Can you work these out from the model? Positions are in its coordinate system, mm. A direction names the side the tool comes from. Give positions to 0.01 mm unless a question says otherwise; leave off trailing zeros. Write each loop counter-clockwise with the first axis right and the second up, starting at its lowest first coordinate (ties: lowest second). Pieces come first, ordered by that corner, then holes.
```python
from build123d import *

# Parameters (mm, degrees)
SKETCH_R        = 2
SKETCH_R_2      = 8.25
SKETCH_R_3      = 3
SKETCH_R_4      = 1.5
PAD_DEPTH       = 10
SKETCH004_R     = 3.5
SKETCH004_R_2   = 2.8
POCKET_DEPTH    = 4
POCKET001_DEPTH = 2.5
SKETCH006_R     = 5
POCKET002_DEPTH = 6


with BuildPart() as part:
    # Sketch → Pad (new body)
    with BuildSketch(Plane.XY):
        with BuildLine():
            Line((0, 0), (0, 34))
            ThreePointArc((0, 34), (-1.757359, 38.242641), (-6, 40))
            Line((-19, 40), (-6, 40))
            ThreePointArc((-25, 46), (-23.242641, 41.757359), (-19, 40))
            Line((-25, 54), (-25, 46))
            ThreePointArc((-19, 60), (-23.242641, 58.242641), (-25, 54))
            Line((-19, 60), (54, 60))
            ThreePointArc((60, 54), (58.242641, 58.242641), (54, 60))
            Line((60, 54), (60, 46))
            ThreePointArc((60, 46), (61.757359, 41.757359), (66, 40))
            Line((66, 40), (89, 40))
            ThreePointArc((95, 34), (93.242641, 38.242641), (89, 40))
            Line((95, 34), (95, 26))
            ThreePointArc((95, 26), (96.757359, 21.757359), (101, 20))
            Line((101, 20), (134, 20))
            ThreePointArc((140, 14), (138.242641, 18.242641), (134, 20))
            Line((140, 14), (140, 0))
            Line((140, 0), (0, 0))
        make_face()
        with Locations((10, 10)):
            Circle(SKETCH_R, mode=Mode.SUBTRACT)
        with Locations((33.5, 39)):
            Circle(SKETCH_R_2, mode=Mode.SUBTRACT)
        with Locations((81.5, 26)):
            Circle(SKETCH_R_3, mode=Mode.SUBTRACT)
        with Locations((130, 10)):
            Circle(SKETCH_R, mode=Mode.SUBTRACT)
        with Locations((40, 10)):
            Circle(SKETCH_R_4, mode=Mode.SUBTRACT)
        with Locations((90, 10)):
            Circle(SKETCH_R_4, mode=Mode.SUBTRACT)
        with Locations((-15.5, 50)):
            Circle(SKETCH_R_3, mode=Mode.SUBTRACT)
    extrude(amount=PAD_DEPTH)

    # Sketch004 → Pocket (cut)
    with BuildSketch(Plane.XY):
        with Locations((10, 10)):
            Circle(SKETCH004_R)
        with Locations((40, 10)):
            Circle(SKETCH004_R_2)
        with Locations((130, 10)):
            Circle(SKETCH004_R)
        with Locations((90, 10)):
            Circle(SKETCH004_R_2)
    extrude(amount=POCKET_DEPTH, mode=Mode.SUBTRACT)

    # Sketch005 (on Face5 of Pocket) → Pocket001 (cut)
    with BuildSketch(Plane.XY.offset(10)):
        Polygon((40, 6.8), (42.771281, 8.4), (42.771281, 11.6), (40, 13.2), (37.228719, 11.6), (37.228719, 8.4), align=None)
        Polygon((90, 6.8), (92.771281, 8.4), (92.771281, 11.6), (90, 13.2), (87.228719, 11.6), (87.228719, 8.4), align=None)
    extrude(amount=-POCKET001_DEPTH, mode=Mode.SUBTRACT)

    # Sketch006 (on Face5 of Pocket) → Pocket002 (cut)
    with BuildSketch(Plane.XY.offset(10)):
        with Locations((81.5, 26)):
            Circle(SKETCH006_R)
        with Locations((-15.5, 50)):
            Circle(SKETCH006_R)
    extrude(amount=-POCKET002_DEPTH, mode=Mode.SUBTRACT)


solid = part.part
```
1) Suppose I cut it at B-B on y = 50. Write out the boundary of the cut face in (x, z).
Values follow:
outline: (-25, 0) - (-18.5, 0) - (-18.5, 4) - (-20.5, 4) - (-20.5, 10) - (-25, 10) - close; (-12.5, 0) - (60, 0) - (60, 10) - (-10.5, 10) - (-10.5, 4) - (-12.5, 4) - close
2) Suppose I cut it at D-D on y = 10. State how many separate pieces and enclosed holes the cut face has, plus the area to 3 significant figures.
Values follow:
separate pieces: 5
enclosed holes: 0
area: 1,200 mm2
3) Suppose I cut it at C-C on z = 1.75. Write out the boundary of the cut face in (x, y).
Values follow:
outline: (-25, 46) arc R6 ccw to (-19, 40) - (-6, 40) arc R6 cw to (0, 34) - (0, 0) - (140, 0) - (140, 14) arc R6 ccw to (134, 20) - (101, 20) arc R6 cw to (95, 26) - (95, 34) arc R6 ccw to (89, 40) - (66, 40) arc R6 cw to (60, 46) - (60, 54) arc R6 ccw to (54, 60) - (-19, 60) arc R6 ccw to (-25, 54) - close; hole circle Ø6 at (-15.5, 50); hole circle Ø7 at (10, 10); hole circle Ø16.5 at (33.5, 39); hole circle Ø5.6 at (40, 10); hole circle Ø6 at (81.5, 26); hole circle Ø5.6 at (90, 10); hole circle Ø7 at (130, 10)
4) Suppose I cut it at A-A on x = 10. Write out the boundary of the cut face in (y, z).
Values follow:
outline: (0, 0) - (6.5, 0) - (6.5, 4) - (8, 4) - (8, 10) - (0, 10) - close; (12, 4) - (13.5, 4) - (13.5, 0) - (60, 0) - (60, 10) - (12, 10) - close
5) Please list where these lines run through material, in increasing order: L1, parallel to Y at x = -15.5, z = 6.75; L2, parallel to X at y = 54, z = 9; L3, parallel to X at y = 11, z = 1.25.
Values follow:
L1: y = 40 to 45, 55 to 60
L2: x = -25 to -18.5, -12.5 to 60
L3: x = 0 to 6.65, 13.35 to 37.38, 42.62 to 87.38, 92.62 to 126.65, 133.35 to 140
6) For pin 1 Ø0.8 at (y, z) = (10.5, 8.5) entering from -X; pin 2 Ø3 at (x, y) = (82.5, 25) entering from +Z; pin 3 Ø1.7 at (x, y) = (39.5, 9.5) entering from -Z; pin 4 Ø3 at (x, y) = (-16, 48) entering from +Z, each with a flat end and sliding along its axis, tell me the tip position at first contact or that it passes through.
Values follow:
pin 1: stops at x = 0
pin 2: passes through
pin 3: stops at z = 4
pin 4: stops at z = 4
7) If we mould it in two halves opening along Y, with no side actions, what happens to faces 1 (the face through (140, 7, 5)), 2 (the face through (58.289, 58.196, 4.93)), 3 (the face through (-13, 40, 5)), 4 (the face through (132, 8, 4))? For each: +Y half, -Y half, draft (parallel to the pull), parting line (faces both ways), or undercut.
Values follow:
face 1: draft
face 2: +Y half
face 3: -Y half
face 4: undercut
8) For faces 5 (the face through (91.2, 8.8, 4)), 6 (the face through (0, 17, 5)), 7 (the face through (32.43, 47.18, 4.93)), 8 (the face through (117, 20, 5)), 9 (the face through (38.7, 8.6, 7.5)), which set-ups out of +Z, -Z, +X, -X, +Y, -Y let a thin tool reach every point of the face, with its end or its side?
Values follow:
face 5: -Z
face 6: +Z, -Z, -X, -Y
face 7: +Z, -Z
face 8: +Z, -Z, +X, +Y
face 9: +Z
